Here's how the part is built. I have some questions about the finished solid (model axes, mm). A direction names the side the tool comes from. Coordinates: 2 decimals unless noted, no trailing zeros. Write each loop counter-clockwise with the first axis right and the second up, starting at its lowest first coordinate (ties: lowest second). Pieces come first, ordered by that corner, then holes.
Item 1: For faces 4 (the face through (0, 2, 2)), 5 (the face through (0.182, 14.715, 4.199)), 6 (the face through (-7.725, 7.107, 4.357)), which set-ups out of +Z, -Z, +X, -X, +Y, -Y let a thin tool reach every point of the face, with its end or its side?
Item 2: I'm going to push flat-ended pins straight in: pin 1 Ø0.8 at (x, z) = (-4, 2) entering from -Y; pin 2 Ø2 at (x, y) = (0, 10) entering from -Z; pin 3 Ø1 at (y, z) = (11, 1) entering from +X. Where does each tip first touch, or does it pass through?
Item 3: If we section it at A-A (z = 3.1): Please give me the cut outline in (x, y).
Item 4: If I drill on line 1 (Z direction, x = 8.5, y = 7.5); line 2 (Y direction, x = 0, z = 0.5); line 3 (X direction, y = 9.5, z = 3.05), over which ranges is the centre line in solid material (lowest first)?
Item 5: We'd pull the mould along Y, two halves only. Please class faces 1 (the face through (-0.16, 11.24, 0.51)), 2 (the face through (22.715, 2.465, 4.199)), 3 (the face through (-17.699, 1.715, 2.268)): +Y half, -Y half, draft (parallel to the pull), parting line (faces both ways), or undercut.
from build123d import *

# Parameters (mm, degrees)
PAD_DEPTH       = 4.5
SKETCH002_R     = 1.25
POCKET_DEPTH    = 5
POCKET001_DEPTH = 3.5
FILLET_R        = 10
FILLET001_R     = 1
FILLET002_R     = 0.5


with BuildPart() as part:
    # Sketch → Pad (new body)
    with BuildSketch(Plane.XY):
        Polygon((23, 15), (23, 0), (18, 0), (18, 2), (-18, 2), (-18, 0), (-23, 0), (-23, 15), align=None)
    extrude(amount=PAD_DEPTH)

    # Sketch002 (on Face10 of Pad) → Pocket (cut)
    with BuildSketch(Plane.XY.offset(4.5)):
        with Locations((0, 10)):
            Circle(SKETCH002_R)
    extrude(amount=-POCKET_DEPTH, mode=Mode.SUBTRACT)

    # Sketch003 (on Face5 of Pocket) → Pocket001 (cut)
    with BuildSketch(Plane.XY.offset(4.5)):
        with BuildLine():
            Line((-15.215333, 11.887758), (-0.408, 13.576805))
            ThreePointArc((0.408, 13.576805), (0, 13.6), (-0.408, 13.576805))
            Line((15.215333, 11.887758), (0.408, 13.576805))
            ThreePointArc((15.215333, 8.112242), (16.9, 10), (15.215333, 11.887758))
            Line((0.408, 6.423195), (15.215333, 8.112242))
            ThreePointArc((-0.408, 6.423195), (0, 6.4), (0.408, 6.423195))
            Line((-15.215333, 8.112242), (-0.408, 6.423195))
            ThreePointArc((-15.215333, 11.887758), (-16.9, 10), (-15.215333, 8.112242))
        make_face()
    extrude(amount=-POCKET001_DEPTH, mode=Mode.SUBTRACT)

    # Fillet
    fillet_edges = [part.edges().sort_by_distance(p)[0] for p in [
        (-23, 15, 2.25),
        (23, 15, 2.25),
    ]]
    fillet(fillet_edges, radius=FILLET_R)

    # Fillet001
    fillet001_edges = [part.edges().sort_by_distance(p)[0] for p in [
        (-18, 1, 0),
        (-18, 1, 4.5),
        (0, 2, 4.5),
        (0, 2, 0),
        (18, 1, 4.5),
        (18, 1, 0),
        (-18, 2, 2.25),
        (18, 2, 2.25),
        (23, 2.5, 4.5),
        (20.071068, 12.071068, 4.5),
        (-20.071068, 12.071068, 4.5),
        (0, 15, 4.5),
        (-23, 2.5, 4.5),
        (23, 2.5, 0),
        (20.071068, 12.071068, 0),
        (0, 15, 0),
        (-20.071068, 12.071068, 0),
        (-23, 2.5, 0),
    ]]
    fillet(fillet001_edges, radius=FILLET001_R)

    # Fillet002
    fillet002_edges = [part.edges().sort_by_distance(p)[0] for p in [
        (-16.9, 10, 4.5),
        (-7.811667, 7.267718, 4.5),
        (0, 6.4, 4.5),
        (7.811667, 7.267718, 4.5),
        (16.9, 10, 4.5),
        (7.811667, 12.732282, 4.5),
        (0, 13.6, 4.5),
        (-7.811667, 12.732282, 4.5),
    ]]
    fillet(fillet002_edges, radius=FILLET002_R)


solid = part.part
Answer list:
1. face 4: +Z, -Z, -Y
1. face 5: +Z, +X, -X, +Y
1. face 6: +Z
2. pin 1: stops at y = 2
2. pin 2: passes through
2. pin 3: stops at x = 21.35
3. outline: (-23, 0) - (-18, 0) - (-18, 1) arc R1 cw to (-17, 2) - (17, 2) arc R1 cw to (18, 1) - (18, 0) - (23, 0) - (23, 5) arc R10 ccw to (13, 15) - (-13, 15) arc R10 ccw to (-23, 5) - close; hole (-15.22, 8.11) - (-0.41, 6.42) arc R3.6 ccw to (0.41, 6.42) - (15.22, 8.11) arc R1.9 ccw to (15.22, 11.89) - (0.41, 13.58) arc R3.6 ccw to (-0.41, 13.58) - (-15.22, 11.89) arc R1.9 ccw to start
4. line 1: z = 0 to 1
4. line 2: y = 2.13 to 8.75, 11.25 to 14.87
4. line 3: x = -21.93 to -16.83, 16.83 to 21.93
5. face 1: undercut
5. face 2: draft
5. face 3: -Y half
